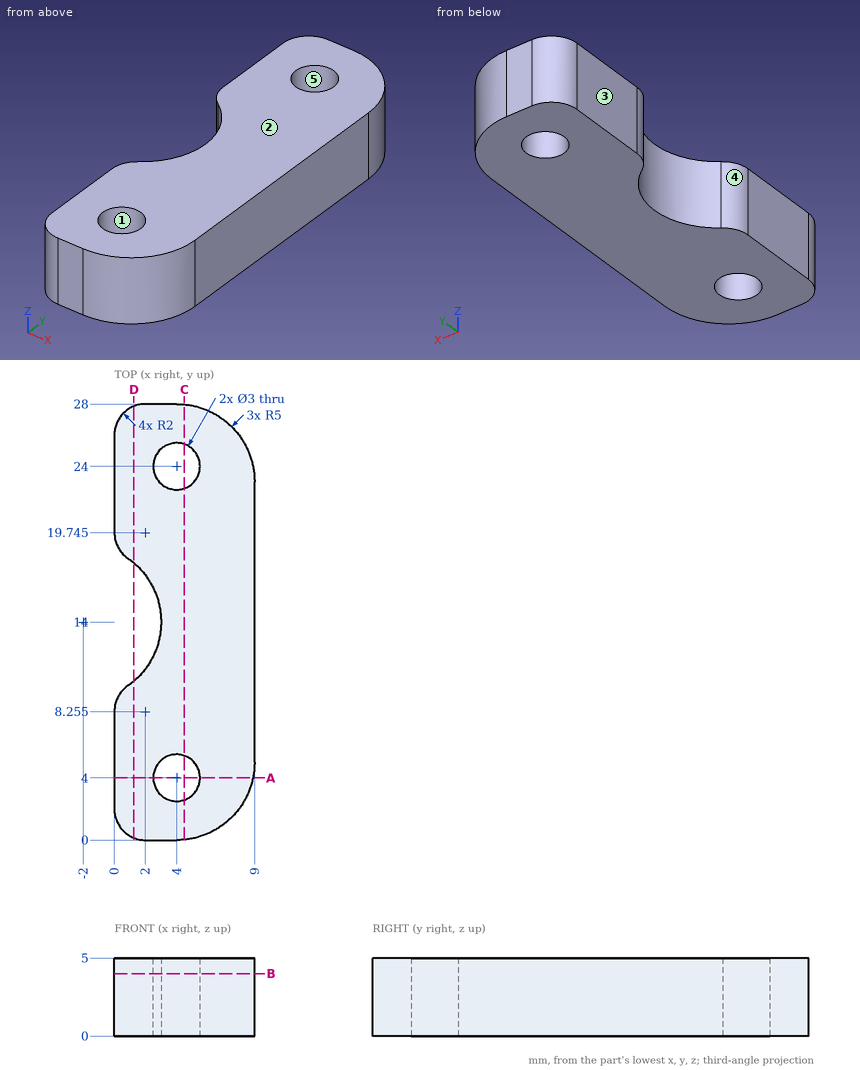
Answer from the drawing. Dimensions are ordinates in mm from the lowest x, y and z of the part. A direction names the side the tool comes from. Round coordinates to 2 decimals unless told otherwise and drop trailing zeros. Write each loop counter-clockwise with the first axis right and the second up, starting at its lowest first coordinate (ties: lowest second). Pieces come first, ordered by that corner, then holes. Notation, with made-up numbers: M 35.5,86.25 L 74.5,86.25 A9 cw 74.5,96.25 Z; hole C -4,64 d1. An arc over 180 degrees is marked long. Write each question's results on one line, items separated by ' | '. Start each with the question number.
Item 1: Straight lines are drawn through the part: probe 1 along X at (y, z) = (4, 2.45); probe 2 along Y at (x, z) = (1, 3.55); probe 3 along Y at (x, z) = (4.25, 2.2). For each, find the intervals that lie inside material, in ascending order.
Item 2: Find section D-D on x = 1.25. Write down the section's boundary in (y, z).
Item 3: The mould has two halves that part along X. Classify the marked faces 1, 2 and 3: +X half, -X half, draft (parallel to the pull), parting line (faces both ways), or undercut.
Item 4: Find section C-C on x = 4.5. Write down the section's boundary in (y, z) (1 decimal).
Item 5: Find section B-B on z = 4. Write down the section's boundary in (x, y) (1 decimal).
Item 6: Find section A-A on y = 4. Write down the section's boundary in (x, z).
Item 7: Which of the six approach directions +Z, -Z, +X, -X, +Y, -Y give full straight-line access (tool end or side, diameter ignored) to the marked faces 4 and 5?
Answer block:
1) probe 1: x = 0 to 2.5, 5.5 to 8.9 | probe 2: y = 0.27 to 10, 18 to 27.73 | probe 3: y = 0.01 to 2.52, 5.48 to 22.52, 25.48 to 27.99
2) outline: M 0.15,0 L 10.2,0 L 10.2,5 L 0.15,5 Z; M 17.8,0 L 27.85,0 L 27.85,5 L 17.8,5 Z
3) face 1: undercut | face 2: draft | face 3: -X half
4) outline: M 0,0 L 2.6,0 L 2.6,5 L 0,5 Z; M 5.4,0 L 22.6,0 L 22.6,5 L 5.4,5 Z; M 25.4,0 L 28,0 L 28,5 L 25.4,5 Z
5) outline: M 0,2 A2 ccw 2,0 L 4,0 A5 ccw 9,5 L 9,23 A5 ccw 4,28 L 2,28 A2 ccw 0,26 L 0,19.7 A2 ccw 0.9,18.1 A5 cw 0.9,9.9 A2 ccw 0,8.3 Z; hole C 4,4 d3; hole C 4,24 d3
6) outline: M 0,0 L 2.5,0 L 2.5,5 L 0,5 Z; M 5.5,0 L 8.9,0 L 8.9,5 L 5.5,5 Z
7) face 4: +Z, -Z, -X | face 5: +Z, -Z
